Autodesk Inventor part; units mm, degrees
ref_plane "YZ Plane" through (0, 0, 0) normal (1, 0, 0) x (0, 1, 0)
ref_plane "XZ Plane" through (0, 0, 0) normal (0, 1, 0) x (-1, 0, 0)
ref_plane "XY Plane" through (0, 0, 0) normal (0, 0, 1) x (1, 0, 0)
sketch "Sketch1" plane through (0, 0, 0) normal (1, 0, 0) x (0, 1, 0)
  line L0 (90.5542, 74.5762) -> (-23.7458, 74.5762)
  line L1 (-23.7458, 74.5762) -> (-23.7458, 49.1762)
  line L2 (-23.7458, 49.1762) -> (90.5542, 49.1762)
  line L3 (90.5542, 49.1762) -> (90.5542, 74.5762)
  line L4 (-23.7458, 66.6387) -> (-26.9208, 66.6387)
  line L5 (-26.9208, 66.6387) -> (-26.9208, 57.1137)
  line L6 (-26.9208, 57.1137) -> (-23.7458, 57.1137)
  line L7 (-23.7458, 57.1137) -> (-23.7458, 66.6387)
  point P0 (0, 0)
  dimension "d0" = 25.4
  dimension "d1" = 114.3
  dimension "d4" = 3.175
  dimension "d5" = 7.9375
  dimension "d6" = 7.9375
extrude "Extrusion2" add sketch "Sketch1" along normal blind 3.175
sketch "Sketch4" plane through (3.175, 0, 0) normal (1, 0, 0) x (0, 0, -1)
  line L0 (-49.1762, 90.5542) -> (-74.5762, 90.5542)
  line L1 (-66.6387, 90.5542) -> (-57.1137, 90.5542)
  line L2 (-57.1137, 90.5542) -> (-57.1137, 87.3792)
  line L3 (-57.1137, 87.3792) -> (-66.6387, 87.3792)
  line L4 (-66.6387, 87.3792) -> (-66.6387, 90.5542)
  line L5 (-49.1762, -23.7458) -> (-49.1762, 90.5542)
  line L6 (-74.5762, 90.5542) -> (-74.5762, -23.7458)
  line L7 (-74.5762, -11.0458) -> (-71.4012, -11.0458)
  line L8 (-71.4012, -11.0458) -> (-71.4012, -1.5208)
  line L9 (-71.4012, -1.5208) -> (-74.5762, -1.5208)
  line L10 (-74.5762, -1.5208) -> (-74.5762, -11.0458)
  line L11 (-74.5762, -23.7458) -> (-66.6387, -23.7458)
  line L12 (-74.5762, 11.1792) -> (-71.4012, 11.1792)
  line L13 (-71.4012, 11.1792) -> (-71.4012, 20.7042)
  line L14 (-71.4012, 20.7042) -> (-74.5762, 20.7042)
  line L15 (-74.5762, 20.7042) -> (-74.5762, 11.1792)
  line L16 (-74.5762, 33.4042) -> (-71.4012, 33.4042)
  line L17 (-71.4012, 33.4042) -> (-71.4012, 42.9292)
  line L18 (-71.4012, 42.9292) -> (-74.5762, 42.9292)
  line L19 (-74.5762, 42.9292) -> (-74.5762, 33.4042)
  line L20 (-71.4012, 55.6292) -> (-74.5762, 55.6292)
  line L21 (-74.5762, 55.6292) -> (-74.5762, 65.1542)
  line L22 (-74.5762, 65.1542) -> (-71.4012, 65.1542)
  line L23 (-71.4012, 65.1542) -> (-71.4012, 55.6292)
  line L24 (-71.4012, 77.8542) -> (-74.5762, 77.8542)
  line L25 (-74.5762, 77.8542) -> (-74.5762, 87.3792)
  line L26 (-74.5762, 87.3792) -> (-71.4012, 87.3792)
  line L27 (-71.4012, 87.3792) -> (-71.4012, 77.8542)
  line L28 (-49.1762, -23.7458) -> (-52.3512, -23.7458)
  line L29 (-52.3512, -23.7458) -> (-52.3512, -11.0458)
  line L30 (-52.3512, -11.0458) -> (-49.1762, -11.0458)
  line L31 (-49.1762, -11.0458) -> (-49.1762, -23.7458)
  line L32 (-49.1762, -1.5208) -> (-52.3512, -1.5208)
  line L33 (-52.3512, -1.5208) -> (-52.3512, 11.1792)
  line L34 (-52.3512, 11.1792) -> (-49.1762, 11.1792)
  line L35 (-49.1762, 11.1792) -> (-49.1762, -1.5208)
  line L36 (-49.1762, 20.7042) -> (-52.3512, 20.7042)
  line L37 (-52.3512, 20.7042) -> (-52.3512, 33.4042)
  line L38 (-52.3512, 33.4042) -> (-49.1762, 33.4042)
  line L39 (-49.1762, 33.4042) -> (-49.1762, 20.7042)
  line L40 (-49.1762, 42.9292) -> (-52.3512, 42.9292)
  line L41 (-52.3512, 42.9292) -> (-52.3512, 55.6292)
  line L42 (-52.3512, 55.6292) -> (-49.1762, 55.6292)
  line L43 (-49.1762, 55.6292) -> (-49.1762, 42.9292)
  line L44 (-49.1762, 65.1542) -> (-52.3512, 65.1542)
  line L45 (-52.3512, 65.1542) -> (-52.3512, 77.8542)
  line L46 (-52.3512, 77.8542) -> (-49.1762, 77.8542)
  line L47 (-49.1762, 77.8542) -> (-49.1762, 65.1542)
  line L48 (-49.1762, 87.3792) -> (-52.3512, 87.3792)
  line L49 (-52.3512, 87.3792) -> (-52.3512, 90.5542)
  line L50 (-52.3512, 90.5542) -> (-49.1762, 90.5542)
  line L51 (-49.1762, 90.5542) -> (-49.1762, 87.3792)
  point P0 (0, 0)
  dimension "d30" = 3.175
  dimension "d31" = 7.9375
  dimension "d32" = 7.9375
  dimension "d33" = 3.175
  dimension "d34" = 9.525
  dimension "d35" = 12.7
  dimension "d36" = 9.525
  dimension "d37" = 12.7
  dimension "d38" = 9.525
  dimension "d39" = 12.7
  dimension "d40" = 9.525
  dimension "d41" = 12.7
  dimension "d42" = 12.7
  dimension "d43" = 9.525
  dimension "d44" = 3.175
extrude "Extrusion5" cut sketch "Sketch4" against normal blind 3.175 contours L5 L48 L49 L0 | L5 L28 L29 L30 | L5 L32 L33 L34 | L5 L36 L37 L38 | L5 L40 L41 L42 | L5 L44 L45 L46 | L9 L8 L7 L6 | L14 L13 L12 L6 | L18 L17 L16 L6 | L22 L23 L20 L6 | L26 L27 L24 L6
The listing builds one solid part. Answer for the finished solid, in the listing's coordinates (mm). A direction names the side the tool comes from. Give positions to 0.01 mm unless a question says otherwise; leave off trailing zeros. Order: outer loops, then holes, each group sorted by start corner. A loop starts at its lowest first (then second) coordinate and runs counter-clockwise, first axis right, second up. Notation, with made-up numbers: (31.5, 85.5) -> (78.5, 85.5) arc R10 cw to (78.5, 103.5) -> close; hole circle Ø4 at (79.25, 3). An arc over 180 degrees is marked (long way). Put each result on its own line as item: value.
Item 1: For faces 1 (the face through (2, 89, 52.351)), 2 (the face through (2, 65.154, 51)), 3 (the face through (2, 20.704, 73)), determine the directions among +Z, -Z, +X, -X, +Y, -Y from which every point of the face is accessible in a straight line to the end or side of a thin tool.
Established:
face 1: -Z, +X, -X, +Y
face 2: -Z, +X, -X
face 3: +Z, +X, -X
Item 2: A cutting plane is placed at A-A on z = 67.75. Give the vertices of the cut face in (x, y) (3 decimals).
Established:
outline: (0, -23.746) -> (3.175, -23.746) -> (3.175, 90.554) -> (0, 90.554) -> close
Item 3: A cutting plane is placed at B-B on y = 39. Give the vertices of the cut face in (x, z) (3 decimals), plus the area to 3 significant figures.
Established:
outline: (0, 49.176) -> (3.175, 49.176) -> (3.175, 71.401) -> (0, 71.401) -> close
area: 70.6 mm^2
Item 4: Given P1, Ø1, axis at x = 1, z = 51, coming from the -Y side; P2, Ø1.6, axis at x = 2, y = 83.5, coming from the +Z side; P3, Ø1, axis at x = 2, z = 73.5, coming from the -Y side, each flat-ended and moving along its own axis, determine where each tip first touches the part or whether it passes through.
Established:
P1: stops at y = -11.05
P2: stops at z = 71.4
P3: stops at y = -23.75
Item 5: For a pull along Y with two mould halves and no side action, classify faces 4 (the face through (2, 5, 74.576)), 5 (the face through (2, -26.921, 62)), 6 (the face through (2, 27, 52.351)), 7 (the face through (2, 55.629, 73)) as released by +Y, released by -Y, zero draft, split by the parting line, or undercut.
Established:
face 4: zero draft
face 5: released by -Y
face 6: undercut
face 7: undercut
Item 6: Straight lines are drawn through the part: line 1 (Y direction, x = 0.45, z = 51.5); line 2 (Y direction, x = 2.3, z = 71.5); line 3 (Z direction, x = 2.4, y = 84.5). For each, find the intervals that lie inside material, in ascending order.
Established:
line 1: y = -11.05 to -1.52, 11.18 to 20.7, 33.4 to 42.93, 55.63 to 65.15, 77.85 to 87.38
line 2: y = -23.75 to -11.05, -1.52 to 11.18, 20.7 to 33.4, 42.93 to 55.63, 65.15 to 77.85, 87.38 to 90.55
line 3: z = 49.18 to 71.4
